```python
from build123d import *

# Parameters (mm, degrees)
SKETCH1_W              = 500
SKETCH1_H              = 210.49
BOSS_EXTRUDE1_DEPTH    = 12
SKETCH2_W              = 83.333333333
SKETCH2_H              = 12
SKETCH2_W_2            = 12
CUT_EXTRUDE1_DEPTH     = 543.632509255
SKETCH3_W              = 12
SKETCH3_H              = 43.245
CUT_EXTRUDE2_DEPTH     = 543.632509255
SCALE1_SCALE           = 0.5
F_12_0MM_DOWEL_SLOT1_D = 12
M4_CLEARANCE_SLOT1_D   = 4.3
F_1_0MM_DOWEL_SLOT1_D  = 30


with BuildPart() as part:
    # Sketch1 → Boss-Extrude1 (new body)
    with BuildSketch(Plane(origin=(0, 0, 0), x_dir=(1, 0, 0), z_dir=(0, 1, 0))):
        with Locations((250, 105.245)):
            Rectangle(SKETCH1_W, SKETCH1_H)
    extrude(amount=BOSS_EXTRUDE1_DEPTH)

    # Sketch2 → Cut-Extrude1 (cut, through all)
    with BuildSketch(Plane(origin=(0, 12, 0), x_dir=(1, 0, 0), z_dir=(0, 1, 0))):
        with Locations((458.333333334, 6)):
            Rectangle(SKETCH2_W, SKETCH2_H)
        with Locations((494, 204.49)):
            Rectangle(SKETCH2_W_2, SKETCH2_H)
        with Locations((6, 204.49)):
            Rectangle(SKETCH2_W_2, SKETCH2_H)
        with Locations((41.666666666, 6)):
            Rectangle(SKETCH2_W, SKETCH2_H)
    extrude(amount=-CUT_EXTRUDE1_DEPTH, mode=Mode.SUBTRACT)

    # Sketch3 → Cut-Extrude2 (cut, through all)
    with BuildSketch(Plane(origin=(0, 12, 0), x_dir=(1, 0, 0), z_dir=(0, 1, 0))):
        with Locations((494, 33.6225)):
            Rectangle(SKETCH3_W, SKETCH3_H)
        with Locations((494, 176.8675)):
            Rectangle(SKETCH3_W, SKETCH3_H)
        with Locations((6, 176.8675)):
            Rectangle(SKETCH3_W, SKETCH3_H)
        with Locations((6, 33.6225)):
            Rectangle(SKETCH3_W, SKETCH3_H)
    extrude(amount=-CUT_EXTRUDE2_DEPTH, mode=Mode.SUBTRACT)


with BuildPart() as part_1:
    # Scale1: scaled about (250, 6, -106.929232272)
    add(part.part.scale(SCALE1_SCALE).moved(Location((125, 3, -53.464616136))))

    # Ø12.0mm Dowel Slot1 (through all)
    with Locations(Plane(origin=(0, 9, 0), x_dir=(1, 0, 0), z_dir=(0, 1, 0))):
        with Locations((188.5, 109.409616136)):
            Hole(F_12_0MM_DOWEL_SLOT1_D / 2)

    # M4 Clearance Slot1 (through all)
    with Locations(Plane(origin=(0, 3, 0), x_dir=(-1, 0, 0), z_dir=(0, -1, 0))):
        with Locations((-188.5, 152.109616136), (-188.5, 66.709616136)):
            Hole(M4_CLEARANCE_SLOT1_D / 2)

    # Ø1.0mm Dowel Slot1 (through all)
    with Locations(Plane(origin=(0, 9, 0), x_dir=(1, 0, 0), z_dir=(0, 1, 0))):
        with Locations((275.228318114, 88.480271571), (335, 93.709616136), (303.604577311, 108.349542167), (272.209154622, 122.989468197), (331.980836508, 128.218812762)):
            Hole(F_1_0MM_DOWEL_SLOT1_D / 2)


solid = part_1.part
```
Build history of the part. All positions in model axes, mm. A direction names the side the tool comes from. Round coordinates to 2 decimals unless told otherwise and drop trailing zeros. Loops run counter-clockwise (first coordinate to the right, second up) from the corner with the lowest first, then second, coordinate; pieces in that order, holes last. Notation, with made-up numbers: M 22,84 L 57,84 A23 cw 57,120 Z; hole C 62.25,-19.5 d2. An arc over 180 degrees is marked long. Answer as CSV lines item,"result".
1. Flat gauge pins, fed straight in: P1, Ø5, axis at x = 191.5, z = -114, coming from the -Y side; P2, Ø1.8, axis at y = 4.5, z = -71, coming from the -X side; P3, Ø3, axis at x = 349.5, y = 6, coming from the +Z side; P4, Ø18, axis at x = 272.21, z = -122.99, coming from the +Y side. Where does each tip first touch, or does it go through?
Resolved:
P1,"stops at y = 3"
P2,"stops at x = 131"
P3,"stops at z = -59.46"
P4,"passes through"
2. Wall check: probe 1 along Z at (x, y) = (188.5, 4.7); probe 2 along Z at (x, y) = (337, 4.05); probe 3 along X at (y, z) = (8.3, -93). Give the ranges that are in metal, low to high. Write a range as [from, to].
Resolved:
probe 1,"z = [-158.71, -154.26], [-149.96, -115.41], [-103.41, -68.86], [-64.56, -53.46]"
probe 2,"z = [-158.71, -142.35], [-114.08, -108.58], [-78.84, -59.46]"
probe 3,"x = [125, 260.93], [289.53, 320.02], [349.98, 375]"
3. Cut at C-C on x = 313.5. Write the cut outline in (y, z).
Resolved:
outline,"M 3,-158.71 L 9,-158.71 L 9,-119.62 L 3,-119.62 Z; M 3,-97.08 L 9,-97.08 L 9,-53.46 L 3,-53.46 Z"
4. Cut at D-D on x = 155. Write the cut outline in (y, z), then the cut area to 3 significant figures.
Resolved:
outline,"M 3,-158.71 L 9,-158.71 L 9,-59.46 L 3,-59.46 Z"
area,"595 mm²"
5. Two-plate mould, pull along Z, no slides. Class faces 5 (the cylindrical face through (343.036, 5.958, -138.357)), 6 (the cylindrical face through (321.144, 5.958, -87.965)), 7 (the flat face through (128, 6, -131.087)), 8 (the flat face through (248, 3, -107)): released by +Z, released by -Z, zero draft, split by the parting line, or undercut.
Resolved:
face 5,"undercut"
face 6,"undercut"
face 7,"released by -Z"
face 8,"zero draft"
6. Cut at A-A on x = 269. Write the cut outline in (y, z).
Resolved:
outline,"M 3,-158.71 L 9,-158.71 L 9,-137.64 L 3,-137.64 Z; M 3,-108.34 L 9,-108.34 L 9,-102.13 L 3,-102.13 Z; M 3,-74.83 L 9,-74.83 L 9,-53.46 L 3,-53.46 Z"
7. 3-axis set-ups, long thin cutter, end or side, ignore diameter. For faces 1 (the flat face through (333.333, 6, -56)), 2 (the flat face through (369, 6, -145)), 3 (the flat face through (166.667, 6, -56)), 4 (the flat face through (131, 6, -145)): which of +Z, -Z, +X, -X, +Y, -Y reach the whole face in a straight line?
Resolved:
face 1,"+Z, +X, +Y, -Y"
face 2,"-Z, +X, +Y, -Y"
face 3,"+Z, -X, +Y, -Y"
face 4,"-Z, -X, +Y, -Y"
8. Cut at B-B on y = 6.8. Count the separate pieces of the cut face and the enclosed holes in it, then the cut area to 3 significant figures.
Resolved:
separate pieces,"1"
enclosed holes,"8"
area,"21,500 mm²"
